from build123d import *

# Parameters (mm, degrees)
BOSS_EXTRUDE1_DEPTH     = 9
SKETCH2_R               = 41.3
SKETCH3_R               = 25.4
SKETCH4_R               = 19
CUT_EXTRUDE1_DEPTH      = 12.6
SKETCH5_R               = 3.2
CUT_EXTRUDE2_DEPTH      = 9
CUT_EXTRUDE3_DEPTH      = 72.824508369
CUT_EXTRUDE3_DEPTH_BACK = 72.824508369
CUT_EXTRUDE4_DEPTH      = 72.824508439


with BuildPart() as part:
    # Sketch1 → Boss-Extrude1 (new body)
    with BuildSketch(Plane.XY):
        with BuildLine():
            Line((-42, 50), (42, 50))
            ThreePointArc((42, 50), (47.656854249, 47.656854249), (50, 42))
            Line((50, 42), (50, -42))
            ThreePointArc((50, -42), (47.656854249, -47.656854249), (42, -50))
            Line((42, -50), (-42, -50))
            ThreePointArc((-42, -50), (-47.656854249, -47.656854249), (-50, -42))
            Line((-50, -42), (-50, 42))
            ThreePointArc((-50, 42), (-47.656854249, 47.656854249), (-42, 50))
        make_face()
    extrude(amount=BOSS_EXTRUDE1_DEPTH)

    # Sketch2 → Loft1 section 0
    with BuildSketch(Plane.XY.offset(9)):
        Circle(SKETCH2_R)
    # Sketch3 → Loft1 section 1
    with BuildSketch(Plane.XY.offset(21.6)):
        Circle(SKETCH3_R)
    loft()

    # Sketch4 → Cut-Extrude1 (cut)
    with BuildSketch(Plane.XY.offset(21.6)):
        Circle(SKETCH4_R)
    extrude(amount=-CUT_EXTRUDE1_DEPTH, mode=Mode.SUBTRACT)

    # Sketch5 → Cut-Extrude2 (cut)
    with BuildSketch(Plane.XY.offset(9)):
        with Locations((-42, 42)):
            Circle(SKETCH5_R)
        with Locations((42, 42)):
            Circle(SKETCH5_R)
    cut_extrude2 = extrude(amount=-CUT_EXTRUDE2_DEPTH, mode=Mode.SUBTRACT)

    # Mirror1: Cut-Extrude2 across plane
    add(cut_extrude2.mirror(Plane.ZX), mode=Mode.SUBTRACT)

    # Sketch6 → Cut-Extrude3 (cut, two sides: drawn at the far end of the back side and taken through both)
    with BuildSketch(Plane.XY.offset(9).offset(-CUT_EXTRUDE3_DEPTH_BACK)):
        with BuildLine():
            Line((-19, -50), (19, -50))
            ThreePointArc((19, -50), (0, -31), (-19, -50))
        make_face()
        with BuildLine():
            Line((-19, 50), (19, 50))
            ThreePointArc((19, 50), (0, 31), (-19, 50))
        make_face()
    extrude(amount=CUT_EXTRUDE3_DEPTH + CUT_EXTRUDE3_DEPTH_BACK, mode=Mode.SUBTRACT)

    # Sketch8 → Cut-Extrude4 (cut, symmetric)
    with BuildSketch(Plane.XY.offset(9)):
        with BuildLine():
            Line((50, 19), (50, -19))
            ThreePointArc((50, -19), (31, 0), (50, 19))
        make_face()
    cut_extrude4 = extrude(amount=CUT_EXTRUDE4_DEPTH, both=True, mode=Mode.SUBTRACT)

    # Mirror3: Cut-Extrude4 across plane
    add(cut_extrude4.mirror(Plane(origin=(0, 0, 0), x_dir=(0, 0, 1), z_dir=(1, 0, 0))), mode=Mode.SUBTRACT)


solid = part.part
Here's how the part is built. I have some questions about the finished solid (model axes, mm). A direction names the side the tool comes from. Round coordinates to 2 decimals unless told otherwise and drop trailing zeros. Write each loop counter-clockwise with the first axis right and the second up, starting at its lowest first coordinate (ties: lowest second). Pieces come first, ordered by that corner, then holes. Notation, with made-up numbers: (18, -0.5) -> (70, -0.5) arc R18 cw to (70, 12.5) -> close; hole circle Ø11 at (32.5, 16.5). An arc over 180 degrees is marked (long way). One line per item, written item: value.
1) I'm going to push flat-ended pins straight in: pin 1 Ø10 at (y, z) = (-17.5, 17.5) entering from +X; pin 2 Ø1.5 at (x, y) = (-14.5, 32) entering from +Z; pin 3 Ø17.5 at (x, y) = (-28.5, -41) entering from +Z; pin 4 Ø1.5 at (x, y) = (-14.5, 19) entering from -Z. Where does each tip first touch, or does it pass through?
Filled sheet:
pin 1: stops at x = 32.91
pin 2: stops at z = 14.48
pin 3: stops at z = 9.09
pin 4: stops at z = 0
2) Suppose I cut it at B-B on z = 15.75. List the corners of the cut face in (x, y) for me, plus the area to 3 significant figures.
Filled sheet:
outline: (-32.14, -6.47) arc R32.78 ccw to (-6.47, -32.14) arc R19 cw to (6.47, -32.14) arc R32.78 ccw to (32.14, -6.47) arc R19 cw to (32.14, 6.47) arc R32.78 ccw to (6.47, 32.14) arc R19 cw to (-6.47, 32.14) arc R32.78 ccw to (-32.14, 6.47) arc R19 cw to start; hole circle Ø38 at (0, 0)
area: 2,180 mm2
3) Suppose I cut it at A-A on x = 0. List the corners of the cut face in (y, z) for me.
Filled sheet:
outline: (-31, 0) -> (31, 0) -> (31, 17.16) -> (25.4, 21.6) -> (19, 21.6) -> (19, 9) -> (-19, 9) -> (-19, 21.6) -> (-25.4, 21.6) -> (-31, 17.16) -> close
4) For faces 1 (the face through (-31, 50, 4)), 2 (the face through (-36, 37, 9)), which set-ups out of +Z, -Z, +X, -X, +Y, -Y let a thin tool reach every point of the face, with its end or its side?
Filled sheet:
face 1: +Z, -Z, +X, -X, +Y
face 2: +Z, -X, +Y
5) If I drill on line 1 (X direction, y = -1, z = 13.5); line 2 (Y direction, x = -42, z = 7), over which ranges is the centre line in solid material (lowest first)? Write a range as [from, to].
Filled sheet:
line 1: x = [-31.03, -18.97], [18.97, 31.03]
line 2: y = [-50, -45.2], [-38.8, -17.23], [17.23, 38.8], [45.2, 50]
6) Suppose I cut it at C-C on x = -40.5. List the corners of the cut face in (y, z) for me.
Filled sheet:
outline: (-50, 0) -> (-44.83, 0) -> (-44.83, 9) -> (-50, 9) -> close; (-39.17, 0) -> (-16.45, 0) -> (-16.45, 9) -> (-39.17, 9) -> close; (16.45, 0) -> (39.17, 0) -> (39.17, 9) -> (16.45, 9) -> close; (44.83, 0) -> (50, 0) -> (50, 9) -> (44.83, 9) -> close
7) We'd pull the mould along X, two halves only. Please class faces 3 (the face through (41.583, 45.173, 4.563)), 4 (the face through (31, -50, 4)), 5 (the face through (-47.719, 47.594, 4.437)), 6 (the face through (24.176, -10.024, 20.988)): released by +X, released by -X, zero draft, split by the parting line, or undercut.
Filled sheet:
face 3: undercut
face 4: zero draft
face 5: released by -X
face 6: split by the parting line
